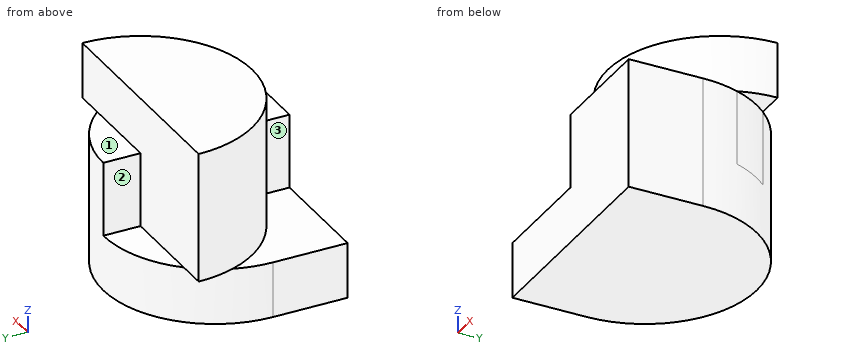
from build123d import *

# Parameters (mm, degrees)
BOSS_EXTRUDE7_DEPTH      = 3.5
SKETCH12_W               = 3
SKETCH12_H               = 2
CUT_EXTRUDE5_DEPTH       = 5.5
BOSS_EXTRUDE8_DEPTH      = 1.5
BOSS_EXTRUDE8_DEPTH_BACK = 2
CUT_EXTRUDE6_DEPTH       = 2


with BuildPart() as part:
    # Sketch11 → Boss-Extrude7 (new body)
    with BuildSketch(Plane.XY):
        with BuildLine():
            Line((3, 0), (3, -2))
            Line((3, -2), (-3, -2))
            Line((-3, -2), (-3, 0))
            ThreePointArc((-3, 0), (0, 3), (3, 0))
        make_face()
    extrude(amount=BOSS_EXTRUDE7_DEPTH)

    # Sketch12 → Cut-Extrude5 (cut)
    with BuildSketch(Plane(origin=(0, -2, 0), x_dir=(-1, 0, 0), z_dir=(0, -1, 0))):
        with Locations((1.5, -2.5)):
            Rectangle(SKETCH12_W, SKETCH12_H)
    extrude(amount=-CUT_EXTRUDE5_DEPTH, mode=Mode.SUBTRACT)

    # Sketch13 → Boss-Extrude8 (add, two sides)
    with BuildSketch(Plane.XY.offset(3.5)) as boss_extrude8_sk:
        with BuildLine():
            Line((-3, 2), (3, 2))
            ThreePointArc((3, 2), (0, -1), (-3, 2))
        make_face()
    extrude(amount=BOSS_EXTRUDE8_DEPTH)
    extrude(boss_extrude8_sk.sketch, amount=-BOSS_EXTRUDE8_DEPTH_BACK)

    # Sketch14 → Cut-Extrude6 (cut)
    with BuildSketch(Plane(origin=(0, 0, 1.5), x_dir=(-1, 0, 0), z_dir=(0, 0, -1))):
        with BuildLine():
            ThreePointArc((-3, 2), (-2.956795679, 1.492694064), (-2.828427125, 1))
            ThreePointArc((-2.828427125, 1), (-2.58113883, 1.528961196), (-2.236067977, 2))
            Line((-2.236067977, 2), (-3, 2))
        make_face()
    extrude(amount=-CUT_EXTRUDE6_DEPTH, mode=Mode.SUBTRACT)


solid = part.part
The model under review builds one solid part; all positions refer to its coordinate system, in mm. Face numbers are marked on the shaded views. A direction names the side the tool comes from. Give positions to 0.01 mm unless a question says otherwise; leave off trailing zeros. Order: outer loops, then holes, each group sorted by start corner. A loop starts at its lowest first (then second) coordinate and runs counter-clockwise, first axis right, second up. Notation, with made-up numbers: M 44.5,87 L 101.5,87 A22 ccw 101.5,116 Z; hole C 28,44 d4. An arc over 180 degrees is marked long. Answer in a Markdown table with one row per item. Add a question column.
1. Add section D-D on x = 1.9. State the section outline as (y, z) points.
2. Add section C-C on y = 1.35. State the section outline as (x, z) points, plus the area to 3 significant figures.
3. Add section A-A on z = 1.8. State the section outline as (x, y) points, plus the area to 3 significant figures.
4. To check wall thickness, follow line 1 along Z through (x, y) = (-1.05, -1.8); line 2 along Z through (x, y) = (2.45, -1.75); line 3 along Y through (x, z) = (-0.1, 0.95). State the ranges of each line that lie inside material, in increasing order.
5. For pin 1 Ø1.1 at (x, y) = (1, 2.5) entering from +Z; pin 2 Ø0.8 at (x, y) = (-0.5, 2.5) entering from +Z; pin 3 Ø1.5 at (x, z) = (1, 3) entering from +Y; pin 4 Ø1 at (y, z) = (1, 2) entering from +X, all flat-tipped, find the tip position at first contact; note any pin that passes through.
6. Add section B-B on x = -0.45. State the section outline as (y, z) points, plus the area to 3 significant figures.
7. Machinability: for the marked faces 1, 2 and 3, which of the approach directions +Z, -Z, +X, -X, +Y, -Y give a long, thin tool a straight path to every point of the face, cutting with its end or side? Answer none if there is none.
The answers:
| question | item | result |
|---|---|---|
| 1 | outline | M -2,0 L 2.32,0 L 2.32,3.5 L 2,3.5 L 2,5 L -0.32,5 L -0.32,3.5 L -2,3.5 Z |
| 2 | outline | M -2.93,1.5 L -2.68,1.5 L -2.68,0 L 2.68,0 L 2.68,3.5 L 2.93,3.5 L 2.93,5 L -2.93,5 Z |
| 2 | area | 28.0 mm2 |
| 3 | outline | M -3,2 A3 ccw 0,-1 L 0,-2 L 3,-2 L 3,0 A3 ccw 0,3 L 0,2 Z |
| 3 | area | 20.1 mm2 |
| 4 | line 1 | 0 to 1.5 |
| 4 | line 2 | 0 to 3.5 |
| 4 | line 3 | -2 to 3 |
| 5 | pin 1 | z = 5 |
| 5 | pin 2 | z = 1.5 |
| 5 | pin 3 | y = 2.99 |
| 5 | pin 4 | x = 2.96 |
| 6 | outline | M -2,0 L 2.97,0 L 2.97,1.5 L 2,1.5 L 2,5 L -0.97,5 L -0.97,1.5 L -2,1.5 Z |
| 6 | area | 17.8 mm2 |
| 7 | face 1 | +Z, +X, -X, +Y |
| 7 | face 2 | +Z, -X, +Y |
| 7 | face 3 | +Z, -X, -Y |
